```python
from build123d import *

# Parameters (mm, degrees)
BOSS_EXTRUDE2_START = -5
BOSS_EXTRUDE2_DEPTH = 9


with BuildPart() as part:
    # Sketch1 → Boss-Extrude2 (new body)
    with BuildSketch(Plane.XY.offset(BOSS_EXTRUDE2_START)):
        with BuildLine():
            ThreePointArc((-14.25, 1), (-17.25, 4), (-14.25, 7))
            Line((-14.25, 7), (-4.833333322, 7))
            ThreePointArc((-4.833333322, 7), (-3, 5.166666661), (-4.833333333, 3.333333333))
            Line((-4.833333333, 3.333333333), (-14.083333333, 3.333333333))
            ThreePointArc((-14.083333333, 3.333333333), (-14.75, 4), (-14.083333333, 4.666666667))
            Line((-14.083333333, 4.666666667), (-4.5, 4.666666667))
            Line((-4.5, 4.666666667), (-4.5, 5.666666667))
            Line((-4.5, 5.666666667), (-14.083333333, 5.666666667))
            ThreePointArc((-14.083333333, 5.666666667), (-15.75, 4), (-14.083333333, 2.333333333))
            Line((-14.083333333, 2.333333333), (-4.833333333, 2.333333333))
            ThreePointArc((-4.833333333, 2.333333333), (-2, 5.166666667), (-4.833333333, 8))
            Line((-4.833333333, 8), (-14.25, 8))
            ThreePointArc((-14.25, 8), (-18.25, 4), (-14.25, 0))
            Line((-14.25, 0), (0, 0))
            Line((0, 0), (0, 1))
            Line((0, 1), (-14.25, 1))
        make_face()
    boss_extrude2 = extrude(amount=BOSS_EXTRUDE2_DEPTH)

    # Mirror1: Boss-Extrude2 across plane
    add(boss_extrude2.mirror(Plane(origin=(0, 0, 0), x_dir=(0, 0, 1), z_dir=(1, 0, 0))))


solid = part.part
```
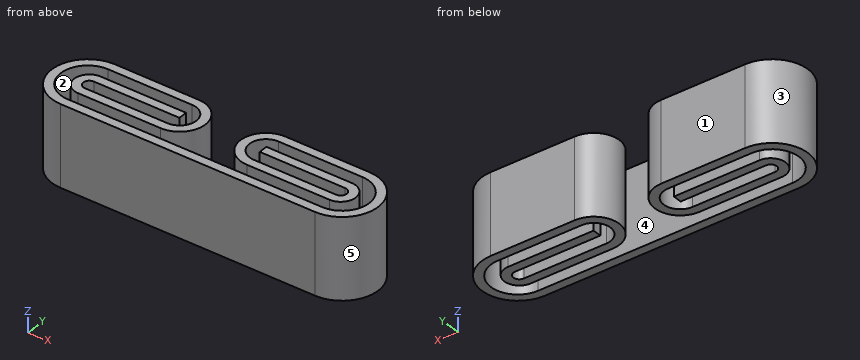
Part model, mm, in its own coordinate system. Face numbers are marked on the shaded views. A direction names the side the tool comes from. Round coordinates to 2 decimals unless told otherwise and drop trailing zeros. Order: outer loops, then holes, each group sorted by start corner. A loop starts at its lowest first (then second) coordinate and runs counter-clockwise, first axis right, second up. Notation, with made-up numbers: M 56.25,-36.5 L 111.25,-36.5 A17 cw 111.25,-25.5 Z; hole C 7.5,60 d5. An arc over 180 degrees is marked long. Put each result on its own line as item: value. Start each with the question number.
1. Slice it at B-B on x = 7. List the corners of the cut face in (y, z).
2. Slice it at A-A on y = 4.25. List the corners of the cut face in (x, z).
3. Drill centre lines: probe 1 along Y at (x, z) = (-6.5, -0.75); probe 2 along X at (y, z) = (3.5, -0.25); probe 3 along Y at (x, z) = (15.5, -2.5). Where is each one in solid material? Low to high. Write a range as [from, to].
4. Drop flat-ended pins along their axis: pin 1 (2.5 mm diameter, centred on x = 2.5, z = 0, fed in from +Y); pin 2 (1 mm diameter, centred on x = 4.5, z = -3.5, fed in from +Y); pin 3 (0.8 mm diameter, centred on y = 5, z = -0.5, fed in from -X); pin 4 (0.5 mm diameter, centred on y = 5, z = -1.5, fed in from +X). Give the stop position or say it passes through.
5. Slice it at C-C on z = -3.25. List the corners of the cut face in (x, y), then the cut area to 3 significant figures.
6. Slice it at D-D on y = 6.25. List the corners of the cut face in (x, z), then the cut area to 3 significant figures.
7. Two-plate mould, pull along Y, no slides. Class the marked faces 1, 2 and 3: +Y half, -Y half, draft (parallel to the pull), parting line (faces both ways), or undercut.
8. Tool access for the marked faces 4 and 5: list every direction of +Z, -Z, +X, -X, +Y, -Y with a clear straight run to the whole face (end or side of a thin tool).
Findings:
1. outline: M 0,-5 L 1,-5 L 1,4 L 0,4 Z; M 2.33,-5 L 3.33,-5 L 3.33,4 L 2.33,4 Z; M 4.67,-5 L 5.67,-5 L 5.67,4 L 4.67,4 Z; M 7,-5 L 8,-5 L 8,4 L 7,4 Z
2. outline: M -18.24,-5 L -17.24,-5 L -17.24,4 L -18.24,4 Z; M -15.73,-5 L -14.7,-5 L -14.7,4 L -15.73,4 Z; M -3.25,-5 L -2.15,-5 L -2.15,4 L -3.25,4 Z; M 2.15,-5 L 3.25,-5 L 3.25,4 L 2.15,4 Z; M 14.7,-5 L 15.73,-5 L 15.73,4 L 14.7,4 Z; M 17.24,-5 L 18.24,-5 L 18.24,4 L 17.24,4 Z
3. probe 1: [0, 1], [2.33, 3.33], [4.67, 5.67], [7, 8]
3. probe 2: [-18.22, -17.21], [-15.67, -14.52], [-4.07, -2.54], [2.54, 4.07], [14.52, 15.67], [17.21, 18.22]
3. probe 3: [0.2, 1.27], [3.12, 4.88], [6.73, 7.8]
4. pin 1: y = 7.78
4. pin 2: y = 8
4. pin 3: x = -18.2
4. pin 4: x = 18.18
5. outline: M -14.25,0 L 14.25,0 A4 ccw 14.25,8 L 4.83,8 A2.83 ccw 4.83,2.33 L 14.08,2.33 A1.67 ccw 14.08,5.67 L 4.5,5.67 L 4.5,4.67 L 14.08,4.67 A0.67 cw 14.08,3.33 L 4.83,3.33 A1.83 cw 4.83,7 L 14.25,7 A3 cw 14.25,1 L -14.25,1 A3 cw -14.25,7 L -4.83,7 A1.83 cw -4.83,3.33 L -14.08,3.33 A0.67 cw -14.08,4.67 L -4.5,4.67 L -4.5,5.67 L -14.08,5.67 A1.67 ccw -14.08,2.33 L -4.83,2.33 A2.83 ccw -4.83,8 L -14.25,8 A4 ccw Z
5. area: 129 mm2
6. outline: M -17.56,-5 L -16.23,-5 L -16.23,4 L -17.56,4 Z; M -3.35,-5 L -2.22,-5 L -2.22,4 L -3.35,4 Z; M 2.22,-5 L 3.35,-5 L 3.35,4 L 2.22,4 Z; M 16.23,-5 L 17.56,-5 L 17.56,4 L 16.23,4 Z
6. area: 44.3 mm2
7. face 1: +Y half
7. face 2: undercut
7. face 3: parting line
8. face 4: +Z, -Z
8. face 5: +Z, -Z, +X
